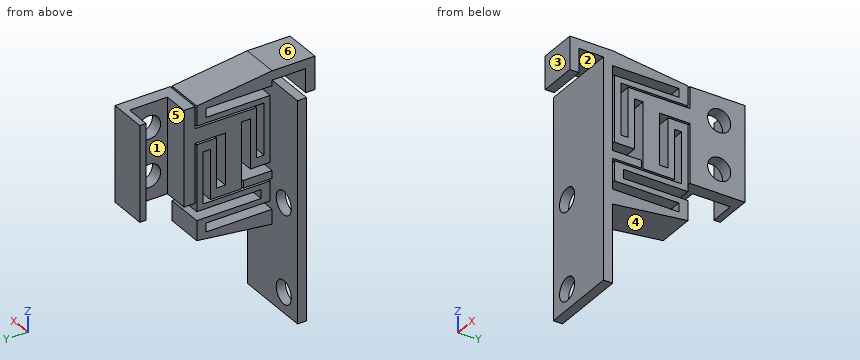
from build123d import *

# Parameters (mm, degrees)
BOSS_EXTRUDE1_DEPTH = 5.18
CUT_EXTRUDE1_REACH  = 33.131
SKETCH2_W           = 3.45
SKETCH2_H           = 5.15
SKETCH3_W           = 10.5
SKETCH3_H           = 30
SKETCH3_R           = 1.575
BOSS_EXTRUDE2_DEPTH = 1.25
CUT_EXTRUDE3_REACH  = 41.726
SKETCH7_R           = 1.575
SKETCH9_W           = 1.05
SKETCH9_H           = 3.9
BOSS_EXTRUDE3_DEPTH = 5.18


with BuildPart() as part:
    # Sketch1 → Boss-Extrude1 (new body)
    with BuildSketch(Plane(origin=(0, 0, 0), x_dir=(0, 0, -1), z_dir=(1, 0, 0))):
        Polygon((0, 0), (13, 0), (13, -7.5), (4.95, -7.5), (4.95, -11.65), (11.95, -11.65), (11.95, -10.45), (5.2, -10.45), (5.2, -7.75), (14.2, -7.75), (14.2, -16.5), (15.4, -16.5), (15.4, -7.75), (18.1, -7.75), (19.35, -18), (19.35, -19.25), (0, -19.25), (0, -22.58), (3.25, -22.58), (3.25, -23.83), (-1.25, -23.83), (-1.25, -18), (0, -7.75), (2.7, -7.75), (2.7, -16.9), (9.7, -16.9), (9.7, -15.9), (2.95, -15.9), (2.95, -7.5), (0, -7.5), align=None)
        Polygon((13.2, -9.6), (13.2, -13.85), (4.2, -13.85), (4.2, -15.05), (10.95, -15.05), (10.95, -17.75), (1.95, -17.75), (1.95, -9), (0.75, -9), (0.75, -18), (17.35, -18), (17.35, -9), (16.15, -9), (16.15, -17.75), (13.45, -17.75), (13.45, -8.6), (6.45, -8.6), (6.45, -9.6), align=None, mode=Mode.SUBTRACT)
    extrude(amount=BOSS_EXTRUDE1_DEPTH)

    # Sketch2 → Cut-Extrude1 (cut, up to next)
    with BuildSketch(Plane.XY, mode=Mode.PRIVATE) as cut_extrude1_sk1:
        with Locations((3.455, -3.425)):
            Rectangle(SKETCH2_W, SKETCH2_H)
    cut_extrude1_tool1 = extrude(cut_extrude1_sk1.sketch, amount=-CUT_EXTRUDE1_REACH, mode=Mode.PRIVATE) & part.part
    add(cut_extrude1_tool1.solids().sort_by_distance((3.455, -3.425, 0))[0], mode=Mode.SUBTRACT)

    # Sketch3 → Boss-Extrude2 (add)
    with BuildSketch(Plane.XZ.offset(19.25)):
        with Locations((5.25, -15)):
            Rectangle(SKETCH3_W, SKETCH3_H)
        with Locations(Location((7.62, -15.23, 0), (0, 0, 270))):
            Circle(SKETCH3_R, mode=Mode.SUBTRACT)
        with Locations(Location((7.62, -27.23, 0), (0, 0, 270))):
            Circle(SKETCH3_R, mode=Mode.SUBTRACT)
    extrude(amount=-BOSS_EXTRUDE2_DEPTH)

    # Sketch7 → Cut-Extrude3 (cut, up to next)
    with BuildSketch(Plane.ZY, mode=Mode.PRIVATE) as cut_extrude3_sk1:
        with Locations((-3.25, -3.5)):
            Circle(SKETCH7_R)
    cut_extrude3_tool1 = extrude(cut_extrude3_sk1.sketch, amount=-CUT_EXTRUDE3_REACH, mode=Mode.PRIVATE) & part.part
    # Sketch7 → Cut-Extrude3 (cut, up to next)
    with BuildSketch(Plane.ZY, mode=Mode.PRIVATE) as cut_extrude3_sk2:
        with Locations((-9.75, -3.5)):
            Circle(SKETCH7_R)
    cut_extrude3_tool2 = extrude(cut_extrude3_sk2.sketch, amount=-CUT_EXTRUDE3_REACH, mode=Mode.PRIVATE) & part.part
    add(cut_extrude3_tool1.solids().sort_by_distance((0, -3.5, -3.25))[0], mode=Mode.SUBTRACT)
    add(cut_extrude3_tool2.solids().sort_by_distance((0, -3.5, -9.75))[0], mode=Mode.SUBTRACT)

    # Sketch9 → Boss-Extrude3 (add)
    with BuildSketch(Plane.ZY):
        with Locations((-12.675, -16.05)):
            Rectangle(SKETCH9_W, SKETCH9_H)
    extrude(amount=-BOSS_EXTRUDE3_DEPTH)


with BuildPart() as body_2:
    # Mirror3: mirrored copy
    add(part.part.mirror(Plane(origin=(0, 0, 0), x_dir=(0, 0, 1), z_dir=(1, 0, 0))))


solid = body_2.part
Could you check a few things on this model? Use its own coordinates, in mm. Face numbers are marked on the shaded views. A direction names the side the tool comes from. Give positions to 0.01 mm unless a question says otherwise; leave off trailing zeros. Loops run counter-clockwise (first coordinate to the right, second up) from the corner with the lowest first, then second, coordinate; pieces in that order, holes last. Notation, with made-up numbers: M 63.25,-24.5 L 115.25,-24.5 A19 cw 115.25,-16.5 Z; hole C -36.5,26.25 d9. An arc over 180 degrees is marked long. Answer as a JSON object with one key per item and string values.
Q1. Suppose I cut it at D-D, the plane y = -11.25. List the corners of the cut face in (x, z) for me.
Values found:
{"outline": "M -5.18,-18.53 L 0,-18.53 L 0,-17.35 L -5.18,-17.35 Z; M -5.18,-16.15 L 0,-16.15 L 0,-15.4 L -5.18,-15.4 Z; M -5.18,-14.2 L 0,-14.2 L 0,-13.45 L -5.18,-13.45 Z; M -5.18,-13.2 L 0,-13.2 L 0,-11.95 L -5.18,-11.95 Z; M -5.18,-4.95 L 0,-4.95 L 0,-2.95 L -5.18,-2.95 Z; M -5.18,-2.7 L 0,-2.7 L 0,-1.95 L -5.18,-1.95 Z; M -5.18,-0.75 L 0,-0.75 L 0,0.43 L -5.18,0.43 Z"}
Q2. Suppose I cut it at B-B, the plane y = -3.5. List the corners of the cut face in (x, z) for me (3 decimals).
Values found:
{"outline": "M -1.73,-13 L 0,-13 L 0,-11.325 L -1.73,-11.325 Z; M -1.73,-8.175 L 0,-8.175 L 0,-4.825 L -1.73,-4.825 Z; M -1.73,-1.675 L 0,-1.675 L 0,0 L -1.73,0 Z"}
Q3. Suppose I cut it at A-A, the plane z = -27.23. List the corners of the cut face in (x, y) for me (3 decimals).
Values found:
{"outline": "M -10.5,-19.25 L -9.195,-19.25 L -9.195,-18 L -10.5,-18 Z; M -6.045,-19.25 L 0,-19.25 L 0,-18 L -6.045,-18 Z"}
Q4. If I drill on probe 1 along Y at (x, z) = (-1.25, -12); probe 2 along Y at (x, z) = (-4.25, -14); probe 3 along Z at (x, y) = (-7.62, -18.3) (3 decimals), over which ranges is the centre line in solid material (lowest first)? Write a range as [from, to].
Values found:
{"probe 1": "y = [-19.25, -18], [-13.85, -9.6], [-8.6, -7.75], [-7.5, 0]", "probe 2": "y = [-19.25, -18], [-17.75, -7.75]", "probe 3": "z = [-30, -28.805], [-25.655, -16.805], [-13.655, 0]"}
Q5. For the marked faces 1, 2 and 3, which set-ups out of +Z, -Z, +X, -X, +Y, -Y let a thin tool reach every point of the face, with its end or its side?
Values found:
{"face 1": "+Z, -Z, -X", "face 2": "-Z, +X, -X", "face 3": "+Z, -Z, +X, -X, -Y"}
Q6. If we mould it in two halves opening along Y, with no side actions, what happens to the marked faces 4, 5 and 6? For each: pulls with the +Y half, pulls with the -Y half, needs draft (parallel to the pull), parting line crosses it, or undercut.
Values found:
{"face 4": "pulls with the +Y half", "face 5": "undercut", "face 6": "needs draft"}
Q7. Suppose I cut it at C-C, the plane x = -2.25. State how many separate pieces and enclosed holes the cut face has, plus the area to 3 significant figures.
Values found:
{"separate pieces": "2", "enclosed holes": "1", "area": "203 mm²"}
Q8. For P1, Ø0.7, axis at y = -0.5, z = -5.5, coming from the -X side; P2, Ø1, axis at y = -20.5, z = -15.5, coming from the +X side; P3, Ø1, axis at x = -3.5, z = -26.5, coming from the +Y side; P4, Ø2, axis at x = -3, y = -9, coming from the +Z side, each with a flat end and sliding along its axis, tell me the tip position at first contact or that it passes through.
Values found:
{"P1": "stops at x = -5.18", "P2": "passes through", "P3": "stops at y = -18", "P4": "stops at z = 0.27"}
